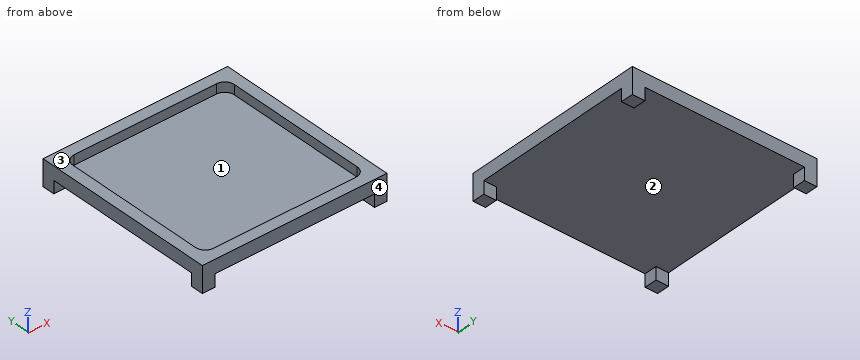
from build123d import *

# Parameters (mm, degrees)
SKETCH1_W           = 96
SKETCH1_H           = 96
BOSS_EXTRUDE1_DEPTH = 2
SKETCH2_W           = 96
SKETCH2_H           = 96
BOSS_EXTRUDE2_DEPTH = 5
SKETCH3_W           = 6.5
SKETCH3_H           = 6.5
BOSS_EXTRUDE3_DEPTH = 6.5


with BuildPart() as part:
    # Sketch1 → Boss-Extrude1 (new body)
    with BuildSketch(Plane.XY):
        Rectangle(SKETCH1_W, SKETCH1_H)
    extrude(amount=BOSS_EXTRUDE1_DEPTH)

    # Sketch2 → Boss-Extrude2 (add)
    with BuildSketch(Plane.XY.offset(2)):
        Rectangle(SKETCH2_W, SKETCH2_H)
        with BuildLine():
            Line((37, -42), (-37, -42))
            ThreePointArc((-37, -42), (-40.535533906, -40.535533906), (-42, -37))
            Line((-42, -37), (-42, 37))
            ThreePointArc((-42, 37), (-40.535533906, 40.535533906), (-37, 42))
            Line((-37, 42), (37, 42))
            ThreePointArc((37, 42), (40.535533906, 40.535533906), (42, 37))
            Line((42, 37), (42, -37))
            ThreePointArc((42, -37), (40.535533906, -40.535533906), (37, -42))
        make_face(mode=Mode.SUBTRACT)
    extrude(amount=BOSS_EXTRUDE2_DEPTH)

    # Sketch3 → Boss-Extrude3 (add)
    with BuildSketch(Plane(origin=(0, 0, 0), x_dir=(-1, 0, 0), z_dir=(0, 0, -1))):
        with Locations((-44.75, 44.75)):
            Rectangle(SKETCH3_W, SKETCH3_H)
        with Locations((44.75, 44.75)):
            Rectangle(SKETCH3_W, SKETCH3_H)
        with Locations((-44.75, -44.75)):
            Rectangle(SKETCH3_W, SKETCH3_H)
        with Locations((44.75, -44.75)):
            Rectangle(SKETCH3_W, SKETCH3_H)
    extrude(amount=BOSS_EXTRUDE3_DEPTH)


solid = part.part
Work out the finished part from the listing and answer in its coordinate system (mm). Face numbers are marked on the shaded views. Give positions to 0.01 mm unless a question says otherwise; leave off trailing zeros. Loops run counter-clockwise (first coordinate to the right, second up) from the corner with the lowest first, then second, coordinate; pieces in that order, holes last. Notation, with made-up numbers: (87.5, 39) -> (96.5, 39) arc R27 ccw to (96.5, 72) -> close; hole circle Ø6 at (-13, -19.75). An arc over 180 degrees is marked (long way). Use a Markdown table: item, result. Add a question column.
1) For a pull along Y with two mould halves and no side action, classify the marked faces 1, 2, 3 and 4 as +Y half, -Y half, draft (parallel to the pull), parting line (faces both ways), or undercut.
2) Consider line 1 along Y through (x, z) = (-21.5, 4); line 2 along Z through (x, y) = (4, 10). Determine where each line is inside the solid, lowest interval first.
3) Each of these flat-tipped pins is pushed along its axis until it touches: P1, Ø1.5, axis at x = 18.5, y = -22, coming from the +Z side; P2, Ø8, axis at x = -22, y = -6.5, coming from the -Z side; P3, Ø5, axis at x = -26, z = -3.5, coming from the -Y side. Where does it stop, or does it pass through?
4) The part is cut by section B-B, the plane y = -32.5. Determine the outline of the cut face in (x, z).
5) The part is cut by section A-A, the plane z = -3. Determine the outline of the cut face in (x, y).
Reported:
| question | item | result |
|---|---|---|
| 1 | face 1 | undercut |
| 1 | face 2 | undercut |
| 1 | face 3 | draft |
| 1 | face 4 | -Y half |
| 2 | line 1 | y = -48 to -42, 42 to 48 |
| 2 | line 2 | z = 0 to 2 |
| 3 | P1 | stops at z = 2 |
| 3 | P2 | stops at z = 0 |
| 3 | P3 | passes through |
| 4 | outline | (-48, 0) -> (48, 0) -> (48, 7) -> (42, 7) -> (42, 2) -> (-42, 2) -> (-42, 7) -> (-48, 7) -> close |
| 5 | outline | (-48, -48) -> (-41.5, -48) -> (-41.5, -41.5) -> (-48, -41.5) -> close; (-48, 41.5) -> (-41.5, 41.5) -> (-41.5, 48) -> (-48, 48) -> close; (41.5, -48) -> (48, -48) -> (48, -41.5) -> (41.5, -41.5) -> close; (41.5, 41.5) -> (48, 41.5) -> (48, 48) -> (41.5, 48) -> close |
